Geometry check sheet. Reference: drawing and pictorial views, mm from the part's lowest x, y, z. A direction names the side the tool comes from. Round coordinates to 2 decimals unless told otherwise and drop trailing zeros. Order: outer loops, then holes, each group sorted by start corner. A loop starts at its lowest first (then second) coordinate and runs counter-clockwise, first axis right, second up.
Q1. Cross-section at D-D on y = 30.5. Record the cut outline in (x, z) (3 decimals), then the cut area to 3 significant figures.
Q2. Set-up check for the marked faces 1 and 2: record each of +Z, -Z, +X, -X, +Y, -Y from which the full face is reachable in a straight line by a thin tool's end or side.
Q3. Cross-section at A-A on x = 139.7. Record the cut outline in (y, z) (3 decimals).
Q4. Cross-section at B-B on y = 94. Record the cut outline in (x, z) (3 decimals), then the cut area to 3 significant figures.
Q5. Scan lines: probe 1 along X at (y, z) = (17, 139.7) (3 decimals); probe 2 along Z at (x, y) = (138.5, 7.5); probe 3 along Y at (x, z) = (108, 21). Record each from-to range of solid material in increasing order.
Q6. Cross-section at C-C on z = 171.5. Record the cut outline in (x, y).
Q7. Depth check by flat-ended pin: P1, Ø2, axis at x = 184.5, y = 22, coming from the -Z side; P2, Ø12, axis at x = 59.5, y = 24, coming from the -Z side; P3, Ø8, axis at x = 89, y = 56.5, coming from the +Z side. Enter the tip coordinate at first touch or a pass-through.
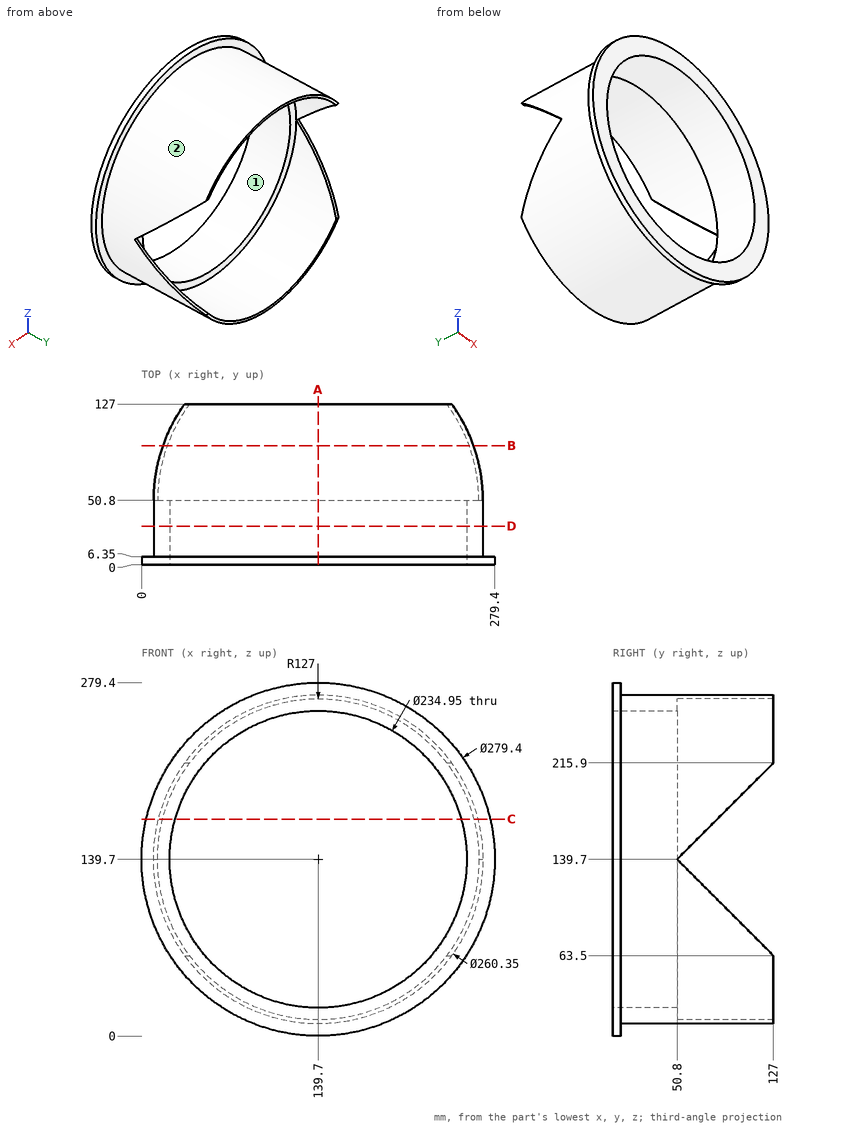
Results found:
1. outline: circle Ø260.35 at (139.7, 139.7); hole circle Ø234.95 at (139.7, 139.7)
1. area: 9,880 mm2
2. face 1: +Y, -Y
2. face 2: +Y
3. outline: (0, 0) - (6.35, 0) - (6.35, 9.525) - (127, 9.525) - (127, 12.7) - (50.8, 12.7) - (50.8, 22.225) - (0, 22.225) - close; (0, 257.175) - (50.8, 257.175) - (50.8, 266.7) - (127, 266.7) - (127, 269.875) - (6.35, 269.875) - (6.35, 279.4) - (0, 279.4) - close
4. outline: (16.902, 96.5) arc R130.175 ccw to (262.498, 96.5) - (259.127, 96.5) arc R127 cw to (20.273, 96.5) - close; (16.902, 182.9) - (20.273, 182.9) arc R127 cw to (259.127, 182.9) - (262.498, 182.9) arc R130.175 ccw to start
4. area: 2,010 mm2
5. probe 1: x = 9.525 to 22.225, 257.175 to 269.875
5. probe 2: z = 9.53 to 22.23, 257.17 to 269.87
5. probe 3: y = 0 to 50.8
6. outline: (3.67, 0) - (26.61, 0) - (26.61, 50.8) - (16.75, 50.8) - (16.75, 82.6) - (13.47, 82.6) - (13.47, 6.35) - (3.67, 6.35) - close; (252.79, 0) - (275.73, 0) - (275.73, 6.35) - (265.93, 6.35) - (265.93, 82.6) - (262.65, 82.6) - (262.65, 50.8) - (252.79, 50.8) - close
7. P1: stops at z = 17.11
7. P2: stops at z = 32.74
7. P3: stops at z = 261.21
